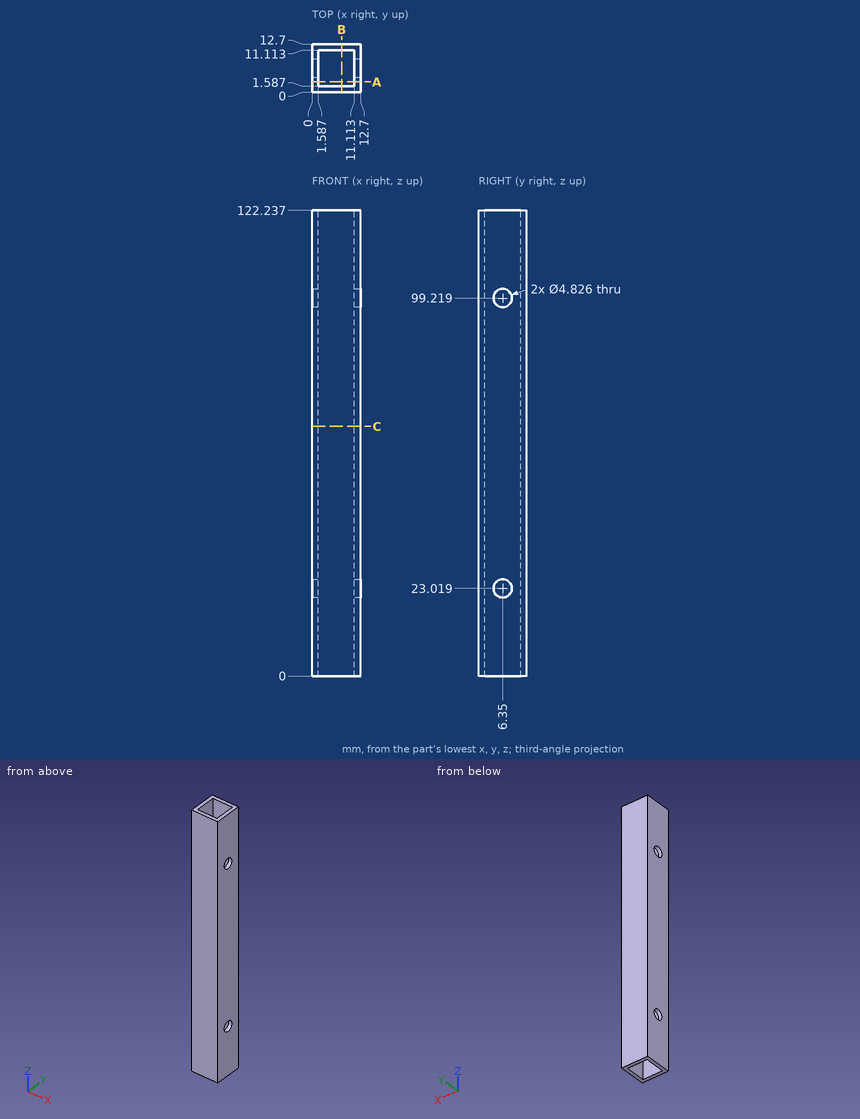
The drawing under review shows one solid part. Ordinate dimensions are in mm from its lowest x, y, z. Round coordinates to 2 decimals unless told otherwise and drop trailing zeros. Write each loop counter-clockwise with the first axis right and the second up, starting at its lowest first coordinate (ties: lowest second). Pieces come first, ordered by that corner, then holes. Notation, with made-up numbers: (39, -4.5) -> (98, -4.5) arc R12 cw to (98, 13.5) -> close; hole circle Ø9 at (54, -6.75). An arc over 180 degrees is marked (long way). Put each result on its own line as item: value.
Q1. To check wall thickness, follow L1, parallel to Z at x = 12.2, y = 6.35 (1 decimal); L2, parallel to Y at x = 3.5, z = 79.5. State the ranges of each line that lie inside material, in increasing order. Write a range as [from, to].
Determined:
L1: z = [0, 20.6], [25.4, 96.8], [101.6, 122.2]
L2: y = [0, 1.59], [11.11, 12.7]
Q2. Consider section C-C on z = 65.5. State the section outline as (x, y) points.
Determined:
outline: (0, 0) -> (12.7, 0) -> (12.7, 12.7) -> (0, 12.7) -> close; hole (1.59, 1.59) -> (11.11, 1.59) -> (11.11, 11.11) -> (1.59, 11.11) -> close
Q3. Clearance check with flat-ended pins moving along their axes: pin 1 Ø3 at (y, z) = (6.35, 99.22) entering from -X; pin 2 Ø2 at (x, z) = (8.5, 24.5) entering from -Y. State where each tip first meets the part, or that it passes through.
Determined:
pin 1: passes through
pin 2: stops at y = 0
Q4. Consider section A-A on y = 2.75. State the section outline as (x, z) points.
Determined:
outline: (0, 0) -> (1.59, 0) -> (1.59, 122.24) -> (0, 122.24) -> close; (11.11, 0) -> (12.7, 0) -> (12.7, 122.24) -> (11.11, 122.24) -> close
